from build123d import *

# Parameters (mm, degrees)
SKETCH5_W           = 395.4
SKETCH5_H           = 265.4
BOSS_EXTRUDE3_DEPTH = 25.4
SKETCH6_W           = 78.175
SKETCH6_H           = 243.175
SKETCH6_W_2         = 75
SKETCH6_H_2         = 240
CUT_EXTRUDE1_DEPTH  = 240.4571778


with BuildPart() as part:
    # Sketch5 → Boss-Extrude3 (new body)
    with BuildSketch(Plane(origin=(0, 0, 0), x_dir=(1, 0, 0), z_dir=(0, 1, 0))):
        Rectangle(SKETCH5_W, SKETCH5_H)
    extrude(amount=BOSS_EXTRUDE3_DEPTH)

    # Sketch6 → Cut-Extrude1 (cut, through all)
    # profile 1 of 4: a face of its own
    with BuildSketch(Plane(origin=(0, 25.4, 0), x_dir=(1, 0, 0), z_dir=(0, 1, 0))):
        with Locations((147.5, 0)):
            Rectangle(SKETCH6_W, SKETCH6_H)
        with Locations((147.5, 0)):
            Rectangle(SKETCH6_W_2, SKETCH6_H_2, mode=Mode.SUBTRACT)
    # profile 2 of 4: a face of its own
    with BuildSketch(Plane(origin=(0, 25.4, 0), x_dir=(1, 0, 0), z_dir=(0, 1, 0))):
        with Locations((147.5, 0)):
            Rectangle(SKETCH6_W_2, SKETCH6_H_2)
    # profile 3 of 4: a face of its own
    with BuildSketch(Plane(origin=(0, 25.4, 0), x_dir=(1, 0, 0), z_dir=(0, 1, 0))):
        with Locations((-147.5, 0)):
            Rectangle(SKETCH6_W, SKETCH6_H)
        with Locations((-147.5, 0)):
            Rectangle(SKETCH6_W_2, SKETCH6_H_2, mode=Mode.SUBTRACT)
    # profile 4 of 4: a face of its own
    with BuildSketch(Plane(origin=(0, 25.4, 0), x_dir=(1, 0, 0), z_dir=(0, 1, 0))):
        with Locations((-147.5, 0)):
            Rectangle(SKETCH6_W_2, SKETCH6_H_2)
    extrude(amount=-CUT_EXTRUDE1_DEPTH, mode=Mode.SUBTRACT)


solid = part.part
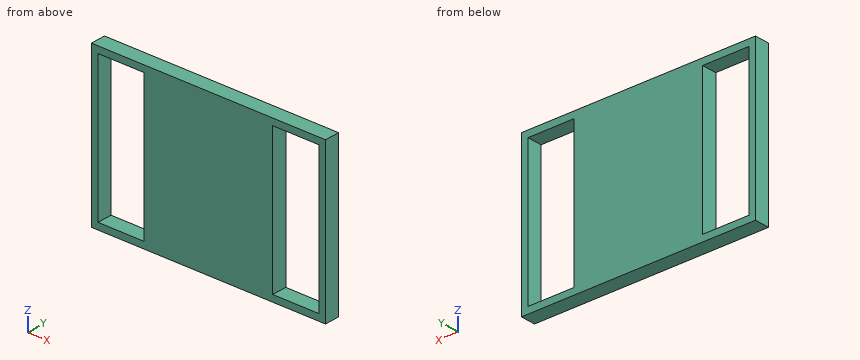
The model under review builds one solid part; all positions refer to its coordinate system, in mm. Coordinates: 2 decimals unless noted, no trailing zeros. Loops run counter-clockwise (first coordinate to the right, second up) from the corner with the lowest first, then second, coordinate; pieces in that order, holes last.
(1) Consider section B-B, the plane y = 14.75. Give the boundary of the cut face in (x, z).
Determined:
outline: (-197.7, -132.7) - (197.7, -132.7) - (197.7, 132.7) - (-197.7, 132.7) - close; hole (-186.59, -121.59) - (-108.41, -121.59) - (-108.41, 121.59) - (-186.59, 121.59) - close; hole (108.41, -121.59) - (186.59, -121.59) - (186.59, 121.59) - (108.41, 121.59) - close
(2) Consider section A-A, the plane z = -19. Give the boundary of the cut face in (x, y), plus the area to 3 significant figures.
Determined:
outline: (-197.7, 0) - (-186.59, 0) - (-186.59, 25.4) - (-197.7, 25.4) - close; (-108.41, 0) - (108.41, 0) - (108.41, 25.4) - (-108.41, 25.4) - close; (186.59, 0) - (197.7, 0) - (197.7, 25.4) - (186.59, 25.4) - close
area: 6,070 mm2
(3) Wall thickness on L1, parallel to X at y = 23, z = 11; L2, parallel to Z at x = -108.5, y = 22.5: over which ranges is each line inside the solid? List them lowest first.
Determined:
L1: x = -197.7 to -186.59, -108.41 to 108.41, 186.59 to 197.7
L2: z = -132.7 to -121.59, 121.59 to 132.7
